For this review, use the dimensioned drawing (mm, ordinates from the lowest corner) and the shaded views. Give positions to 0.01 mm unless a question says otherwise; leave off trailing zeros. Loops run counter-clockwise (first coordinate to the right, second up) from the corner with the lowest first, then second, coordinate; pieces in that order, holes last. Notation, with made-up numbers: M 81.5,68.5 L 111.5,68.5 A24 ccw 111.5,102.5 Z; hole C 48.25,12 d8. An arc over 180 degrees is marked long. Return JSON: item names as keys, results as strings.
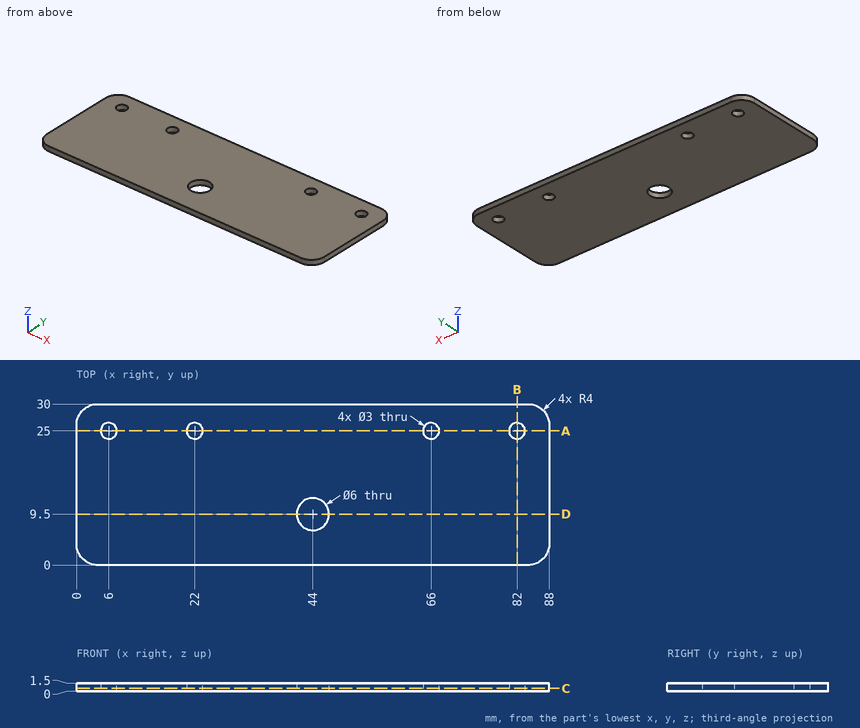
1) Consider section A-A on y = 25. Write out the cut boundary in (x, z), then the cut area to 3 significant figures.
From the geometry:
{"outline": "M 0,0 L 4.5,0 L 4.5,1.5 L 0,1.5 Z; M 7.5,0 L 20.5,0 L 20.5,1.5 L 7.5,1.5 Z; M 23.5,0 L 64.5,0 L 64.5,1.5 L 23.5,1.5 Z; M 67.5,0 L 80.5,0 L 80.5,1.5 L 67.5,1.5 Z; M 83.5,0 L 88,0 L 88,1.5 L 83.5,1.5 Z", "area": "114 mm²"}
2) Consider section B-B on x = 82. Write out the cut boundary in (y, z), then the cut area to 3 significant figures.
From the geometry:
{"outline": "M 0,0 L 23.5,0 L 23.5,1.5 L 0,1.5 Z; M 26.5,0 L 30,0 L 30,1.5 L 26.5,1.5 Z", "area": "40.5 mm²"}
3) Consider section C-C on z = 0.55. Write out the cut boundary in (x, y), then the cut area to 3 significant figures.
From the geometry:
{"outline": "M 0,4 A4 ccw 4,0 L 84,0 A4 ccw 88,4 L 88,26 A4 ccw 84,30 L 4,30 A4 ccw 0,26 Z; hole C 6,25 d3; hole C 22,25 d3; hole C 44,9.5 d6; hole C 66,25 d3; hole C 82,25 d3", "area": "2,570 mm²"}
4) Wall thickness on L1, parallel to Y at x = 44, z = 0.75; L2, parallel to Y at x = 6, z = 1.15; L3, parallel to X at y = 12, z = 1.4: over which ranges is each line inside the solid? List them lowest first. Write a range as from..to.
From the geometry:
{"L1": "0..6.5, 12.5..30", "L2": "0..23.5, 26.5..30", "L3": "0..42.34, 45.66..88"}
5) Consider section D-D on y = 9.5. Write out the cut boundary in (x, z).
From the geometry:
{"outline": "M 0,0 L 41,0 L 41,1.5 L 0,1.5 Z; M 47,0 L 88,0 L 88,1.5 L 47,1.5 Z"}
6) Insertion check: pin 1 (2.5 mm diameter, centred on x = 82, y = 25, fed in from -Z). The pin has a flat end and moves straight along its axis. Give the tip position at first contact, or say it passes through.
From the geometry:
{"pin 1": "through"}
